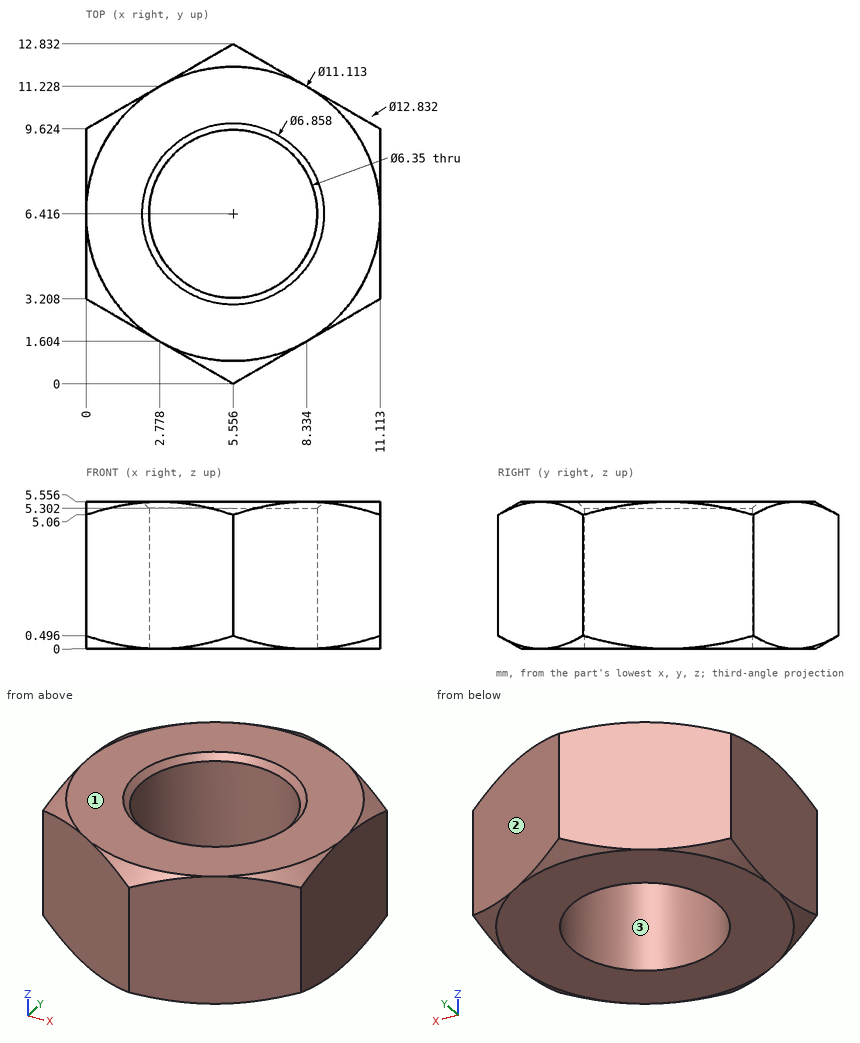
For this review, use the dimensioned drawing (mm, ordinates from the lowest corner) and the shaded views. Round coordinates to 2 decimals unless told otherwise and drop trailing zeros. Write each question's results on one line, items separated by ' | '. Start each with the question number.
1. To check wall thickness, follow L1, parallel to Y at x = 6, z = 1.8 (1 decimal); L2, parallel to Y at x = 4.75, z = 4.4 (1 decimal); L3, parallel to X at y = 4.5, z = 5.2 (1 decimal). State the ranges of each line that lie inside material, in increasing order. Write a range as [from, to].
2. Draft analysis for pull direction Y (two halves, no side actions). For the marked faces 1, 2 and 3, state which applies: pulls with the +Y half, pulls with the -Y half, needs draft (parallel to the pull), parting line crosses it, or undercut.
3. Clearance check with flat-ended pins moving along their axes: pin 1 Ø5.5 at (x, y) = (5.56, 6.42) entering from +Z; pin 2 Ø2 at (x, z) = (3.5, 2.5) entering from -Y; pin 3 Ø2 at (x, z) = (2.5, 3) entering from +Y (1 decimal); pin 4 Ø1.5 at (x, z) = (7, 3.5) entering from +Y. State where each tip first meets the part, or that it passes through.
Output values:
1) L1: [0.3, 3.3], [9.6, 12.6] | L2: [0.5, 3.3], [9.5, 12.4] | L3: [0, 3], [8.1, 11.1]
2) face 1: needs draft | face 2: pulls with the +Y half | face 3: undercut
3) pin 1: through | pin 2: y = 0.61 | pin 3: y = 11.6 | pin 4: y = 12.43
